The listing builds one solid part. Answer for the finished solid, in the listing's coordinates (mm). Round coordinates to 2 decimals unless told otherwise and drop trailing zeros. Write each loop counter-clockwise with the first axis right and the second up, starting at its lowest first coordinate (ties: lowest second). Pieces come first, ordered by that corner, then holes.
Item 1: Find section C-C on z = 2.25. Give the vertices of the cut face in (x, y), then the cut area to 3 significant figures.
Item 2: Find section B-B on x = 22.25. Give the vertices of the cut face in (y, z).
Item 3: Find section A-A on y = 0. Give the vertices of the cut face in (x, z).
Item 4: Find section D-D on y = -4.25. Give the vertices of the cut face in (x, z), then the cut area to 3 significant figures.
Item 5: Find the intervals of material crossed by probe 1 along Y at (x, z) = (-22.25, 0.85); probe 2 along X at (y, z) = (0.5, 2.05); probe 3 along X at (y, z) = (2.25, 2.2), in increasing order.
```python
from build123d import *

# Parameters (mm, degrees)
F1_DEPTH = 3


with BuildPart() as f1:
    # F0 (on Top) → F1 (new body)
    with BuildSketch(Plane.XY):
        with BuildLine():
            Line((-25, -6.5), (25, -6.5))
            ThreePointArc((25, -6.5), (28.535534, -5.035534), (30, -1.5))
            Line((30, -1.5), (30, 0))
            Line((30, 0), (25, 0))
            ThreePointArc((25, 0), (22.25, -2.75), (19.5, 0))
            Line((19.5, 0), (-19.5, 0))
            ThreePointArc((-19.5, 0), (-22.25, -2.75), (-25, 0))
            Line((-25, 0), (-30, 0))
            Line((-30, 0), (-30, -1.5))
            ThreePointArc((-30, -1.5), (-28.535534, -5.035534), (-25, -6.5))
        make_face()
        with BuildLine():
            Line((25, 0), (30, 0))
            Line((30, 0), (30, 1.5))
            ThreePointArc((30, 1.5), (28.535534, 5.035534), (25, 6.5))
            Line((25, 6.5), (-25, 6.5))
            ThreePointArc((-25, 6.5), (-28.535534, 5.035534), (-30, 1.5))
            Line((-30, 1.5), (-30, 0))
            Line((-30, 0), (-25, 0))
            ThreePointArc((-25, 0), (-22.25, 2.75), (-19.5, 0))
            Line((-19.5, 0), (19.5, 0))
            ThreePointArc((19.5, 0), (22.25, 2.75), (25, 0))
        make_face()
    extrude(amount=F1_DEPTH)


solid = f1.part
```
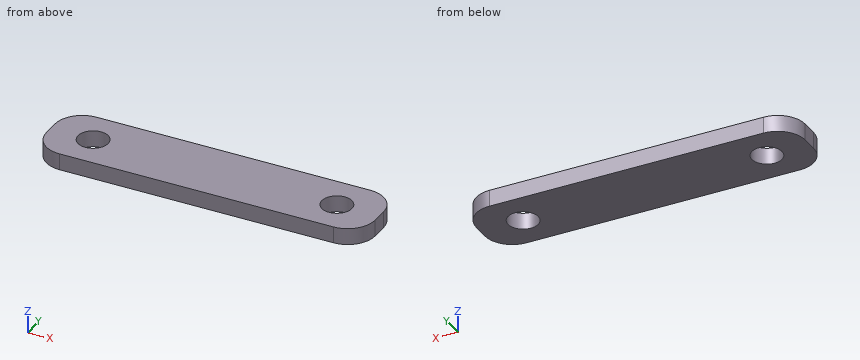
Check values:
1. outline: (-30, -1.5) arc R5 ccw to (-25, -6.5) - (25, -6.5) arc R5 ccw to (30, -1.5) - (30, 1.5) arc R5 ccw to (25, 6.5) - (-25, 6.5) arc R5 ccw to (-30, 1.5) - close; hole circle Ø5.5 at (-22.25, 0); hole circle Ø5.5 at (22.25, 0)
1. area: 711 mm2
2. outline: (-6.5, 0) - (-2.75, 0) - (-2.75, 3) - (-6.5, 3) - close; (2.75, 0) - (6.5, 0) - (6.5, 3) - (2.75, 3) - close
3. outline: (-30, 0) - (-25, 0) - (-25, 3) - (-30, 3) - close; (-19.5, 0) - (19.5, 0) - (19.5, 3) - (-19.5, 3) - close; (25, 0) - (30, 0) - (30, 3) - (25, 3) - close
4. outline: (-29.18, 0) - (29.18, 0) - (29.18, 3) - (-29.18, 3) - close
4. area: 175 mm2
5. probe 1: y = -6.5 to -2.75, 2.75 to 6.5
5. probe 2: x = -30 to -24.95, -19.55 to 19.55, 24.95 to 30
5. probe 3: x = -29.94 to -23.83, -20.67 to 20.67, 23.83 to 29.94
